CAD build for the part. Positions are in the model's coordinates, mm. A direction names the side the tool comes from. Coordinates: 2 decimals unless noted, no trailing zeros. Loops run counter-clockwise (first coordinate to the right, second up) from the corner with the lowest first, then second, coordinate; pieces in that order, holes last.
1) Saw through at C-C, the plane y = 12.25. Write the cut outline in (x, z).
2) Pin check, flat tip, straight feed: pin 1 Ø10 at (x, y) = (8, 14) entering from +Z. Stop position of the tip, or through.
3) Saw through at A-A, the plane y = 2. Write the cut outline in (x, z).
4) Which spindle directions (+Z, -Z, +X, -X, +Y, -Y) get a long thin tool onto all of the face, cutting with end or side? Do faces 1 (the flat face through (10, 0, 5)), 2 (the cylindrical face through (1.2, 1.4, 11)). Say none if no direction does.
5) Wall check: line 1 along Z through (x, y) = (9.75, 16.5). Give the ranges that are in metal, low to high.
```python
from build123d import *

# Parameters (mm, degrees)
SKETCH_1_W     = 20
SKETCH_1_H     = 20
BASEBOX_DEPTH  = 10
SKETCH_2_R     = 1
BOSSSEED_DEPTH = 2


with BuildPart() as part:
    # 草图1 → BaseBox (new body)
    with BuildSketch(Plane.XY):
        with Locations((10, 10)):
            Rectangle(SKETCH_1_W, SKETCH_1_H)
    extrude(amount=BASEBOX_DEPTH)

    # 草图2 → BossSeed (add)
    with BuildSketch(Plane.XY.offset(10)):
        with Locations((2, 2)):
            Circle(SKETCH_2_R)
    extrude(amount=BOSSSEED_DEPTH)


solid = part.part
```
Data:
1. outline: (0, 0) - (20, 0) - (20, 10) - (0, 10) - close
2. pin 1: stops at z = 10
3. outline: (0, 0) - (20, 0) - (20, 10) - (3, 10) - (3, 12) - (1, 12) - (1, 10) - (0, 10) - close
4. face 1: +Z, -Z, +X, -X, -Y
4. face 2: +Z
5. line 1: z = 0 to 10
